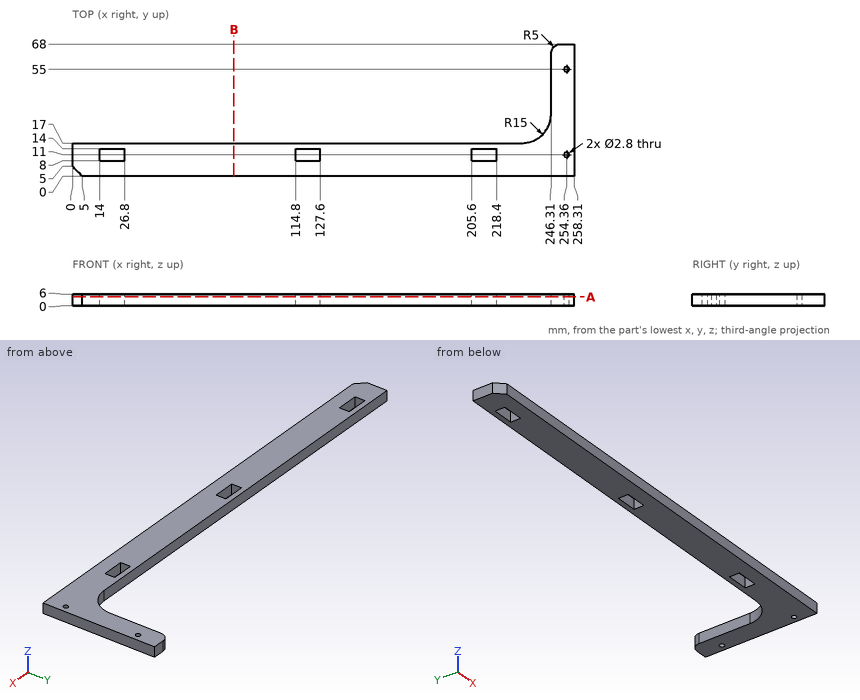
The figure shows three views and two pictorial views of one solid part (mm, origin at its lowest corner). Answer the questions. Round coordinates to 2 decimals unless told otherwise and drop trailing zeros. Write each loop counter-clockwise with the first axis right and the second up, starting at its lowest first coordinate (ties: lowest second). Pieces come first, ordered by that corner, then holes. Notation, with made-up numbers: (35, -5) -> (69, -5) arc R29 ccw to (69, 16) -> close; hole circle Ø2 at (-34, 53.5). An arc over 180 degrees is marked (long way). Answer as a JSON object with one key per item and string values. Group by question number.
Q1. This flat-tipped pin is pushed along its axis until it touches: pin 1 Ø3 at (y, z) = (35.5, 3.5) entering from -X. Where does it stop, or does it pass through?
Q2. Straight lines are drawn through the part: line 1 along Y through (x, z) = (254.36, 2.2); line 2 along Y through (x, z) = (213, 3.35); line 3 along X through (y, z) = (34, 4.9). For each, find the intervals that lie inside material, in ascending order.
Q3. Section A-A (z = 4.6) is taken. Write down the section's boundary in (x, y), plus the area to 3 significant figures.
Q4. Section B-B (x = 83) is taken. Write down the section's boundary in (y, z), plus the area to 3 significant figures.
Check values:
{
 "1": {"pin 1": "x = 246.31"},
 "2": {"line 1": "0 to 9.6, 12.4 to 53.6, 56.4 to 68", "line 2": "0 to 8, 14 to 17", "line 3": "246.31 to 258.31"},
 "3": {"outline": "(0, 5) -> (5, 0) -> (258.31, 0) -> (258.31, 68) -> (251.31, 68) arc R5 ccw to (246.31, 63) -> (246.31, 32) arc R15 cw to (231.31, 17) -> (0, 17) -> close; hole (14, 8) -> (26.8, 8) -> (26.8, 14) -> (14, 14) -> close; hole (114.8, 8) -> (127.6, 8) -> (127.6, 14) -> (114.8, 14) -> close; hole (205.6, 8) -> (218.4, 8) -> (218.4, 14) -> (205.6, 14) -> close; hole circle Ø2.8 at (254.36, 11); hole circle Ø2.8 at (254.36, 55)", "area": "4,790 mm^2"},
 "4": {"outline": "(0, 0) -> (17, 0) -> (17, 6) -> (0, 6) -> close", "area": "102 mm^2"}
}
